```python
from build123d import *

# Parameters (mm, degrees)
SKETCH1_W             = 56
SKETCH1_H             = 34
SKETCH1_W_2           = 52
SKETCH1_H_2           = 30
BASE_DEPTH            = 1.5
SKETCH1_3_W           = 56
SKETCH1_3_H           = 34
SKETCH1_3_W_2         = 52
SKETCH1_3_H_2         = 30
BOSS_EXTRUDE2_DEPTH   = 3
SKETCH2_W             = 53.6
SKETCH2_H             = 31.6
SKETCH2_W_2           = 52
SKETCH2_H_2           = 30
WALL_DEPTH            = 2.3
SKETCH3_W             = 1.2
SKETCH3_H             = 3.75
GROOVEFOROPEN_DEPTH   = 1
LOCKPINS_START        = 13.5
SKETCH4_R             = 0.6
LOCKPINS_DEPTH        = 6
FILLETBASE_R          = 1
FILLETINNER_R         = 0.8
CUTCABLE_DEPTH        = 34.182676203
CUTFORCONNECTOR_DEPTH = 34.182676203


with BuildPart() as part:
    # Sketch1 → Base (new body)
    with BuildSketch(Plane(origin=(0, 0, 0), x_dir=(1, 0, 0), z_dir=(0, 1, 0))):
        Rectangle(SKETCH1_W, SKETCH1_H)
        Rectangle(SKETCH1_W_2, SKETCH1_H_2, mode=Mode.SUBTRACT)
        Rectangle(SKETCH1_W_2, SKETCH1_H_2)
    extrude(amount=BASE_DEPTH)

    # Sketch1_3 → Boss-Extrude2 (add)
    with BuildSketch(Plane(origin=(0, 0, 0), x_dir=(1, 0, 0), z_dir=(0, 1, 0))):
        Rectangle(SKETCH1_3_W, SKETCH1_3_H)
        Rectangle(SKETCH1_3_W_2, SKETCH1_3_H_2, mode=Mode.SUBTRACT)
    extrude(amount=BOSS_EXTRUDE2_DEPTH)

    # Sketch2 → Wall (add)
    with BuildSketch(Plane(origin=(0, 3, 0), x_dir=(1, 0, 0), z_dir=(0, 1, 0))):
        Rectangle(SKETCH2_W, SKETCH2_H)
        Rectangle(SKETCH2_W_2, SKETCH2_H_2, mode=Mode.SUBTRACT)
    extrude(amount=WALL_DEPTH)

    # Sketch3 → GrooveForOpen (cut)
    with BuildSketch(Plane(origin=(0, 3, 0), x_dir=(1, 0, 0), z_dir=(0, 1, 0))):
        with Locations((-27.4, -8.375)):
            Rectangle(SKETCH3_W, SKETCH3_H)
        with Locations((-27.4, 8.375)):
            Rectangle(SKETCH3_W, SKETCH3_H)
    extrude(amount=-GROOVEFOROPEN_DEPTH, mode=Mode.SUBTRACT)

    # Sketch4 → LockPins (add)
    with BuildSketch(Plane(origin=(0, 0, 0), x_dir=(0, 0, -1), z_dir=(1, 0, 0)).offset(LOCKPINS_START)):
        with Locations((15.8, 4.7)):
            Circle(SKETCH4_R)
        with Locations((-15.8, 4.7)):
            Circle(SKETCH4_R)
    lockpins = extrude(amount=LOCKPINS_DEPTH)

    # LockPins2: LockPins across plane
    add(lockpins.mirror(Plane(origin=(0, 0, 0), x_dir=(0, 0, 1), z_dir=(1, 0, 0))))

    # FilletBase
    filletbase_edges = [part.edges().sort_by_distance(p)[0] for p in [
        (0, 0, -17),
        (28, 0, 0),
        (0, 0, 17),
        (-28, 0, 0),
        (-28, 1.5, -17),
        (28, 1.5, -17),
        (28, 1.5, 17),
        (-28, 1.5, 17),
    ]]
    fillet(filletbase_edges, radius=FILLETBASE_R)

    # FilletInner
    filletinner_edges = [part.edges().sort_by_distance(p)[0] for p in [
        (-26.8, 4.15, -15.8),
        (-26.8, 4.15, 15.8),
        (26.8, 4.15, 15.8),
        (26.8, 4.15, -15.8),
    ]]
    fillet(filletinner_edges, radius=FILLETINNER_R)

    # Sketch5 → CutCable (cut, through all)
    with BuildSketch(Plane(origin=(0, 0, 0), x_dir=(0, 0, -1), z_dir=(1, 0, 0))):
        with BuildLine():
            Line((-4.5, 5.462258994), (4.5, 5.462258994))
            Line((4.5, 5.462258994), (4.5, 3.4))
            ThreePointArc((4.5, 3.4), (4.412132034, 3.187867966), (4.2, 3.1))
            Line((4.2, 3.1), (-4.2, 3.1))
            ThreePointArc((-4.2, 3.1), (-4.412132034, 3.187867966), (-4.5, 3.4))
            Line((-4.5, 3.4), (-4.5, 5.462258994))
        make_face()
    extrude(amount=-CUTCABLE_DEPTH, mode=Mode.SUBTRACT)

    # Sketch7 → CutForConnector (cut, through all)
    with BuildSketch(Plane.XZ):
        with BuildLine():
            Line((28.0151422, -5.25), (16.7, -5.25))
            ThreePointArc((16.7, -5.25), (15.992893219, -4.957106781), (15.7, -4.25))
            Line((15.7, -4.25), (15.7, 4.25))
            ThreePointArc((15.7, 4.25), (15.992893219, 4.957106781), (16.7, 5.25))
            Line((16.7, 5.25), (28.0151422, 5.25))
            Line((28.0151422, 5.25), (28.0151422, -5.25))
        make_face()
    extrude(amount=-CUTFORCONNECTOR_DEPTH, mode=Mode.SUBTRACT)


solid = part.part
```
Here's how the part is built. I have some questions about the finished solid (model axes, mm). A direction names the side the tool comes from. Round coordinates to 2 decimals unless told otherwise and drop trailing zeros. Order: outer loops, then holes, each group sorted by start corner. A loop starts at its lowest first (then second) coordinate and runs counter-clockwise, first axis right, second up. Notation, with made-up numbers: (-12, 66.25) -> (31, 66.25) arc R23 cw to (31, 103.25) -> close; hole circle Ø7 at (86.5, 10.25). An arc over 180 degrees is marked (long way). Use a Markdown table: item, result. Add a question column.
(1) Suppose I cut it at A-A, the plane z = 3. Please give me the cut outline in (x, y).
(2) If we mould it in two halves opening along Y, with no side actions, what happens to faces 6 (the face through (0.378, 0.301, 16.715)), 7 (the face through (16.5, 4.7, -16.4)), 8 (the face through (0, 3, -15))? For each: released by +Y, released by -Y, zero draft, split by the parting line, or undercut.
(3) For faces 1 (the face through (26, 3, -10)), 2 (the face through (24, 1, -5.25)), 3 (the face through (-27.4, 2.5, 10.25)), 4 (the face through (-27, 3, 0)), 5 (the face through (26.8, 4, 10)), which set-ups out of +Z, -Z, +X, -X, +Y, -Y let a thin tool reach every point of the face, with its end or its side?
(4) I need wall thicknesses on line 1 along X through (y, z) = (5.15, 11.5); line 2 along Z through (x, y) = (21, 1.4); line 3 along X through (y, z) = (2.9, -9). Which ranges of each line are inside material? Lowest first, please.
(5) For pin 1 Ø1.8 at (y, z) = (4.5, -8) entering from +X; pin 2 Ø1.8 at (x, y) = (-7.5, 4.5) entering from +Z; pin 3 Ø12 at (x, z) = (-7.5, 7) entering from +Y, each with a flat end and sliding along its axis, tell me the tip position at first contact or that it passes through.
(6) Suppose I cut it at C-C, the plane z = 11. Please give me the cut outline in (x, y), and give its area (3 significant figures).
(7) Suppose I cut it at B-B, the plane x = -5. Please give me the cut outline in (y, z), and give its area (3 significant figures).
Verdict:
| question | item | result |
|---|---|---|
| 1 | outline | (-28, 1) arc R1 ccw to (-27, 0) -> (15.7, 0) -> (15.7, 1.5) -> (-26, 1.5) -> (-26, 3.1) -> (-26.8, 3.1) -> (-26.8, 3) -> (-28, 3) -> close |
| 2 | face 6 | released by -Y |
| 2 | face 7 | undercut |
| 2 | face 8 | zero draft |
| 3 | face 1 | +Y |
| 3 | face 2 | +X, +Y, -Y |
| 3 | face 3 | -X, +Y |
| 3 | face 4 | +Z, -Z, -X, +Y |
| 3 | face 5 | +Z, -Z, +X, +Y |
| 4 | line 1 | -26.8 to -26, 26 to 26.8 |
| 4 | line 2 | -17 to -5.25, 5.25 to 17 |
| 4 | line 3 | -26.8 to -26, 26 to 28 |
| 5 | pin 1 | x = 26.8 |
| 5 | pin 2 | z = 15.8 |
| 5 | pin 3 | y = 1.5 |
| 6 | outline | (-28, 1) arc R1 ccw to (-27, 0) -> (27, 0) arc R1 ccw to (28, 1) -> (28, 3) -> (26.8, 3) -> (26.8, 5.3) -> (26, 5.3) -> (26, 1.5) -> (-26, 1.5) -> (-26, 5.3) -> (-26.8, 5.3) -> (-26.8, 3) -> (-28, 3) -> close |
| 6 | area | 93.3 mm2 |
| 7 | outline | (0, -16) arc R1 ccw to (1, -17) -> (3, -17) -> (3, -15.8) -> (5.3, -15.8) -> (5.3, -15) -> (1.5, -15) -> (1.5, 15) -> (5.3, 15) -> (5.3, 15.8) -> (3, 15.8) -> (3, 17) -> (1, 17) arc R1 ccw to (0, 16) -> close |
| 7 | area | 60.3 mm2 |
